Can you work these out from the model? Positions are in its coordinate system, mm. A direction names the side the tool comes from. Give positions to 0.01 mm unless a question says otherwise; leave off trailing zeros. Order: outer loops, then holes, each group sorted by start corner. A loop starts at its lowest first (then second) coordinate and runs counter-clockwise, first axis right, second up. Notation, with made-up numbers: M 60.25,-31 L 76.25,-31 A20 ccw 76.25,-7 Z; hole C -4.75,62.5 d2. An arc over 180 degrees is marked long. Use one line per item in the form item = value. Start each with the question number.
1. I need wall thicknesses on L1, parallel to Z at x = 35, y = 5; L2, parallel to X at y = 57.5, z = 4.5; L3, parallel to Z at x = 58.5, y = 57. Which ranges of each line are inside material? Lowest first, please.
2. We'd pull the mould along X, two halves only. Please class faces 6 (the face through (-45, 10, 0)), 7 (the face through (-55, 20, 0)), 8 (the face through (-40.15, 49, 0)): +X half, -X half, draft (parallel to the pull), parting line (faces both ways), or undercut.
3. I want a section at D-D, the plane y = 11. List the corners of the cut face in (x, z) for me, and give its area (3 significant figures).
4. I want a section at A-A, the plane x = 35. List the corners of the cut face in (y, z) for me, and give its area (3 significant figures).
5. I want a section at C-C, the plane x = -55. List the corners of the cut face in (y, z) for me, and give its area (3 significant figures).
6. For faces 1 (the face through (31, 7, 17)), 2 (the face through (55, 20, 0)), 3 (the face through (53, 60, 0)), 4 (the face through (-40.15, 49, -24)), 5 (the face through (30.904, 17.846, 15.18)), which set-ups out of +Z, -Z, +X, -X, +Y, -Y let a thin tool reach every point of the face, with its end or its side?
7. I want a section at B-B, the plane y = 54. List the corners of the cut face in (x, z) for me.
8. Will these pins go through, and if not, where does the flat tip stop? P1, Ø12, axis at x = -8, z = 9.5, coming from the +Y side; P2, Ø1, axis at y = 13, z = 0, coming from the +X side; P3, Ø5.5, axis at x = -36, z = -18.5, coming from the +Y side.
```python
from build123d import *

# Parameters (mm, degrees)
SKETCH1_W               = 130
SKETCH1_H               = 50
BOSS_EXTRUDE1_DEPTH     = 60
SKETCH2_W               = 80.3
SKETCH2_H               = 40
CUT_EXTRUDE1_DEPTH      = 51
SKETCH3_R               = 4.1
CUT_EXTRUDE2_DEPTH      = 61
SKETCH4_R               = 8
CUT_EXTRUDE3_DEPTH      = 7
CHAMFER1_SIZE           = 1
SKETCH5_OUTSIDE_W       = 162.332
SKETCH5_OUTSIDE_H       = 82.332
SKETCH5_OUTSIDE_W_2     = 90
SKETCH5_OUTSIDE_H_2     = 50
CUT_EXTRUDE4_DEPTH      = 20
SKETCH6_R               = 4.1
CUT_EXTRUDE5_DEPTH      = 41
SKETCH7_R               = 9
CUT_EXTRUDE6_DEPTH      = 21
CUT_EXTRUDE6_DEPTH_BACK = 11


with BuildPart() as part:
    # Sketch1 → Boss-Extrude1 (new body)
    with BuildSketch(Plane(origin=(0, 0, 0), x_dir=(1, 0, 0), z_dir=(0, 1, 0))):
        Rectangle(SKETCH1_W, SKETCH1_H)
    extrude(amount=BOSS_EXTRUDE1_DEPTH)

    # Sketch2 → Cut-Extrude1 (cut, through all)
    with BuildSketch(Plane.XY.offset(25)):
        with Locations((0, 60)):
            Rectangle(SKETCH2_W, SKETCH2_H)
    extrude(amount=-CUT_EXTRUDE1_DEPTH, mode=Mode.SUBTRACT)

    # Sketch3 → Cut-Extrude2 (cut, through all)
    with BuildSketch(Plane.XZ):
        with Locations((-35, 15)):
            Circle(SKETCH3_R)
        with Locations((-35, -15)):
            Circle(SKETCH3_R)
        with Locations((35, -14.217273236)):
            Circle(SKETCH3_R)
        with Locations((35, 15)):
            Circle(SKETCH3_R)
    extrude(amount=-CUT_EXTRUDE2_DEPTH, mode=Mode.SUBTRACT)

    # Sketch4 → Cut-Extrude3 (cut)
    with BuildSketch(Plane.XZ):
        with Locations((35, 15)):
            Circle(SKETCH4_R)
        with Locations((35, -14.217273236)):
            Circle(SKETCH4_R)
        with Locations((-35, 15)):
            Circle(SKETCH4_R)
        with Locations((-35, -15)):
            Circle(SKETCH4_R)
    extrude(amount=-CUT_EXTRUDE3_DEPTH, mode=Mode.SUBTRACT)

    # Chamfer1
    chamfer1_edges = [part.edges().sort_by_distance(p)[0] for p in [
        (40.15, 60, 0),
        (-40.15, 60, 0),
    ]]
    chamfer(chamfer1_edges, length=CHAMFER1_SIZE)

    # Sketch5 outside → Cut-Extrude4 (cut)
    with BuildSketch(Plane.XZ):
        Rectangle(SKETCH5_OUTSIDE_W, SKETCH5_OUTSIDE_H)
        Rectangle(SKETCH5_OUTSIDE_W_2, SKETCH5_OUTSIDE_H_2, mode=Mode.SUBTRACT)
    extrude(amount=-CUT_EXTRUDE4_DEPTH, mode=Mode.SUBTRACT)

    # Sketch6 → Cut-Extrude5 (cut, through all)
    with BuildSketch(Plane.XZ.offset(-20)):
        with Locations((55, -12.5)):
            Circle(SKETCH6_R)
        with Locations((55, 12.5)):
            Circle(SKETCH6_R)
        with Locations((-55, -12.5)):
            Circle(SKETCH6_R)
        with Locations((-55, 12.5)):
            Circle(SKETCH6_R)
    extrude(amount=-CUT_EXTRUDE5_DEPTH, mode=Mode.SUBTRACT)

    # Sketch7 → Cut-Extrude6 (cut, two sides)
    with BuildSketch(Plane(origin=(0, 40, 0), x_dir=(1, 0, 0), z_dir=(0, 1, 0))) as cut_extrude6_sk:
        with Locations((35, -15)):
            Circle(SKETCH7_R)
        with Locations((-35, -15)):
            Circle(SKETCH7_R)
        with Locations((35, 14.217273236)):
            Circle(SKETCH7_R)
        with Locations((-35, 15)):
            Circle(SKETCH7_R)
    extrude(amount=CUT_EXTRUDE6_DEPTH, mode=Mode.SUBTRACT)
    extrude(cut_extrude6_sk.sketch, amount=-CUT_EXTRUDE6_DEPTH_BACK, mode=Mode.SUBTRACT)


solid = part.part
```
Check result:
q1.L1 = -25 to -22.22, -6.22 to 7, 23 to 25
q1.L2 = -65 to -40.15, 40.15 to 65
q1.L3 = -25 to -14.64, -10.36 to 10.36, 14.64 to 25
q2.face_6 = -X half
q2.face_7 = draft
q2.face_8 = undercut
q3.outline = M -45,-25 L 45,-25 L 45,25 L -45,25 Z; hole C -35,-15 d8.2; hole C -35,15 d8.2; hole C 35,-14.22 d8.2; hole C 35,15 d8.2
q3.area = 4,290 mm2
q4.outline = M 0,-25 L 40,-25 L 40,-23.22 L 29,-23.22 L 29,-18.32 L 7,-18.32 L 7,-22.22 L 0,-22.22 Z; M 0,-6.22 L 7,-6.22 L 7,-10.12 L 29,-10.12 L 29,-5.22 L 40,-5.22 L 40,6 L 29,6 L 29,10.9 L 7,10.9 L 7,7 L 0,7 Z; M 0,23 L 7,23 L 7,19.1 L 29,19.1 L 29,24 L 40,24 L 40,25 L 0,25 Z
q4.area = 1,020 mm2
q5.outline = M 20,-25 L 60,-25 L 60,-16.6 L 20,-16.6 Z; M 20,-8.4 L 60,-8.4 L 60,8.4 L 20,8.4 Z; M 20,16.6 L 60,16.6 L 60,25 L 20,25 Z
q5.area = 1,340 mm2
q6.face_1 = -Y
q6.face_2 = +Z, -Z, +X, -Y
q6.face_3 = +Z, -Z, +X, -X, +Y
q6.face_4 = +Z, -Z, +Y
q6.face_5 = +Y, -Y
q7.outline = M -65,-25 L -40.15,-25 L -40.15,-22.38 A9 cw -40.15,-7.62 L -40.15,7.62 A9 cw -40.15,22.38 L -40.15,25 L -65,25 Z; M 40.15,-25 L 65,-25 L 65,25 L 40.15,25 L 40.15,22.38 A9 cw 40.15,7.62 L 40.15,-6.84 A9 cw 40.15,-21.6 Z; hole C -55,-12.5 d8.2; hole C -55,12.5 d8.2; hole C 55,-12.5 d8.2; hole C 55,12.5 d8.2
q8.P1 = 40
q8.P2 = 45
q8.P3 = 29
